Geometry: see drawing. Coordinates: mm, zero at the bounding-box minimum. Give positions to 0.01 mm unless a question says otherwise; leave off trailing zeros. Write each loop counter-clockwise with the first axis right and the second up, starting at its lowest first coordinate (ties: lowest second). Pieces come first, ordered by that corner, then holes. Notation, with made-up numbers: M 60,77 L 80,77 A12 ccw 80,82 Z; hole C 76,68.5 d8. An arc over 180 degrees is marked long. Use a Markdown table: item, result. Add a question column.
(1) Draft query along X for the marked faces 1, 2, 3 and 4. Return one class per face: released by +X, released by -X, zero draft, split by the parting line, or undercut.
(2) Pin query (flat end, axial travel): pin 1 Ø5 at (x, y) = (17.5, 1) entering from +Z; pin 2 Ø4 at (x, y) = (13, 4) entering from -Z. Return the tip coordinate at first contact, or that it passes through.
(3) Cut plane C-C (z = 2.5). Output: boundary loops of the cut face in (x, y).
(4) Material intervals for L1, parallel to X at y = 1, z = 3.3; L2, parallel to Z at x = 22, y = 5.75; L3, parallel to Y at x = 12.5, z = 2.4, sorted ascending.
(5) Cut plane D-D (z = 4.5). Output: boundary loops of the cut face in (x, y).
(6) Cut plane B-B (x = 3). Output: boundary loops of the cut face in (y, z).
(7) Cut plane A-A (y = 1.75). Output: boundary loops of the cut face in (x, z).
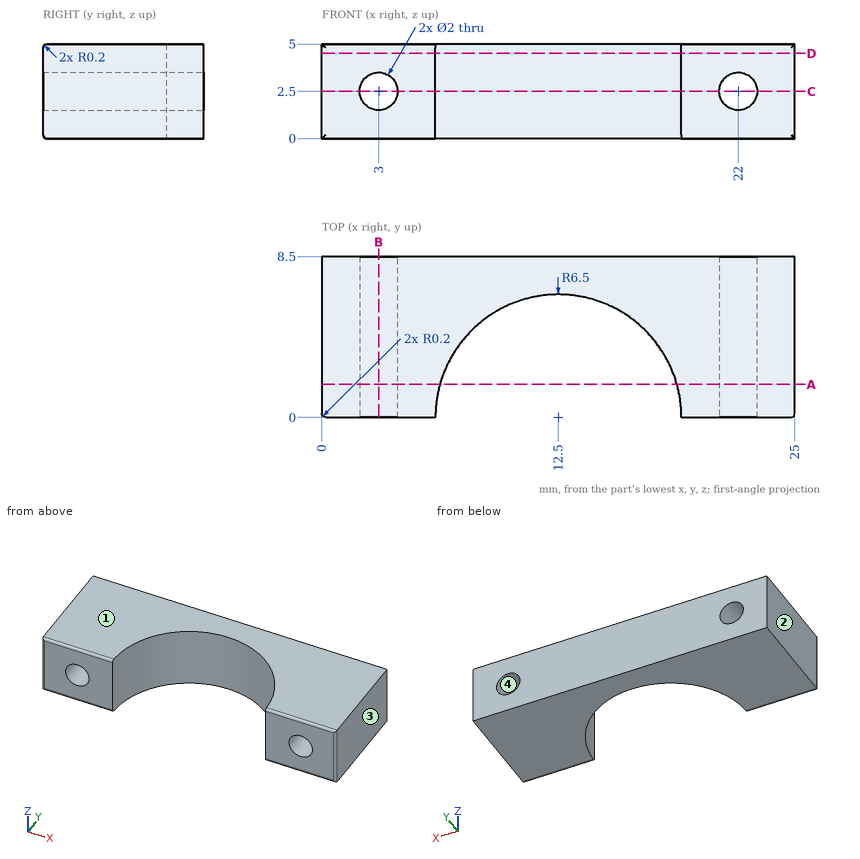
Answer list:
| question | item | result |
|---|---|---|
| 1 | face 1 | zero draft |
| 1 | face 2 | released by -X |
| 1 | face 3 | released by +X |
| 1 | face 4 | undercut |
| 2 | pin 1 | z = 5 |
| 2 | pin 2 | through |
| 3 | outline | M 0,0.2 A0.2 ccw 0.2,0 L 2,0 L 2,8.5 L 0,8.5 Z; M 4,0 L 6,0 A6.5 cw 19,0 L 21,0 L 21,8.5 L 4,8.5 Z; M 23,0 L 24.8,0 A0.2 ccw 25,0.2 L 25,8.5 L 23,8.5 Z |
| 4 | L1 | 0 to 2.4, 3.6 to 6.08, 18.92 to 21.4, 22.6 to 25 |
| 4 | L2 | 0 to 1.5, 3.5 to 5 |
| 4 | L3 | 6.5 to 8.5 |
| 5 | outline | M 0,0.2 A0.2 ccw 0.2,0 L 6,0 A6.5 cw 19,0 L 24.8,0 A0.2 ccw 25,0.2 L 25,8.5 L 0,8.5 Z |
| 6 | outline | M 0,0.2 A0.2 ccw 0.2,0 L 8.5,0 L 8.5,1.5 L 0,1.5 Z; M 0,3.5 L 8.5,3.5 L 8.5,5 L 0.2,5 A0.2 ccw 0,4.8 Z |
| 7 | outline | M 0,0 L 6.24,0 L 6.24,5 L 0,5 Z; M 18.76,0 L 25,0 L 25,5 L 18.76,5 Z; hole C 3,2.5 d2; hole C 22,2.5 d2 |
